from build123d import *

# Parameters (mm, degrees)
SKETCH1_W           = 23
SKETCH1_H           = 60
BOSS_EXTRUDE1_DEPTH = 55
SKETCH2_W           = 55
SKETCH2_H           = 9.5
CUT_EXTRUDE1_DEPTH  = 5
SKETCH3_R           = 1.75
CUT_EXTRUDE2_DEPTH  = 3


with BuildPart() as part:
    # Sketch1 → Boss-Extrude1 (new body)
    with BuildSketch(Plane(origin=(0, 0, 0), x_dir=(0, 0, -1), z_dir=(1, 0, 0))):
        with Locations((11.5, 30)):
            Rectangle(SKETCH1_W, SKETCH1_H)
    extrude(amount=BOSS_EXTRUDE1_DEPTH)

    # Sketch2 → Cut-Extrude1 (cut)
    with BuildSketch(Plane.XY):
        with Locations((27.5, 52.25)):
            Rectangle(SKETCH2_W, SKETCH2_H)
    extrude(amount=-CUT_EXTRUDE1_DEPTH, mode=Mode.SUBTRACT)

    # Sketch3 → Cut-Extrude2 (cut)
    with BuildSketch(Plane.XY.offset(-5)):
        with Locations((7.5, 52.25)):
            Circle(SKETCH3_R)
        with Locations((27.5, 52.25)):
            Circle(SKETCH3_R)
        with Locations((47.5, 52.25)):
            Circle(SKETCH3_R)
    extrude(amount=-CUT_EXTRUDE2_DEPTH, mode=Mode.SUBTRACT)


solid = part.part
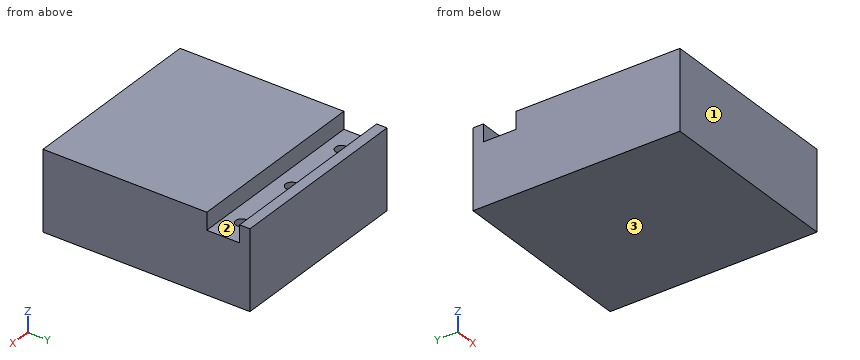
Work out the finished part from the listing and answer in its coordinate system (mm). Face numbers are marked on the shaded views. Round coordinates to 2 decimals unless told otherwise and drop trailing zeros. Write each loop counter-clockwise with the first axis right and the second up, starting at its lowest first coordinate (ties: lowest second). Pieces come first, ordered by that corner, then holes. Notation, with made-up numbers: (33, 58) -> (60, 58) arc R6 ccw to (60, 64) -> close; hole circle Ø2 at (56, 33.5). An arc over 180 degrees is marked (long way). Write each question's results on one line, items separated by ' | '.
Item 1: The mould has two halves that part along Y. Classify the marked faces 1, 2 and 3: +Y half, -Y half, draft (parallel to the pull), parting line (faces both ways), or undercut.
Result set:
face 1: -Y half | face 2: undercut | face 3: draft
Item 2: A cutting plane is placed at A-A, the plane z = -2.75. Determine the outline of the cut face in (x, y).
Result set:
outline: (0, 0) -> (55, 0) -> (55, 47.5) -> (0, 47.5) -> close; (0, 57) -> (55, 57) -> (55, 60) -> (0, 60) -> close
Item 3: A cutting plane is placed at B-B, the plane x = 36. Determine the outline of the cut face in (y, z), plus the area to 3 significant figures.
Result set:
outline: (0, -23) -> (60, -23) -> (60, 0) -> (57, 0) -> (57, -5) -> (47.5, -5) -> (47.5, 0) -> (0, 0) -> close | area: 1,330 mm^2
Item 4: Find the intervals of material crossed by line 1 along Y through (x, z) = (27.5, -5.65); line 2 along Y through (x, z) = (38.5, -2.25), in increasing order. Write a range as [from, to].
Result set:
line 1: [0, 50.5], [54, 60] | line 2: [0, 47.5], [57, 60]
Item 5: A cutting plane is placed at C-C, the plane x = 7.5. Determine the outline of the cut face in (y, z), plus the area to 3 significant figures.
Result set:
outline: (0, -23) -> (60, -23) -> (60, 0) -> (57, 0) -> (57, -5) -> (54, -5) -> (54, -8) -> (50.5, -8) -> (50.5, -5) -> (47.5, -5) -> (47.5, 0) -> (0, 0) -> close | area: 1,320 mm^2
Item 6: Flat-ended cylindrical pins translate along their axes: P1, Ø1.5, axis at x = 7.5, z = -14, coming from the -Y side; P2, Ø1, axis at x = 8, y = 52, coming from the +Z side; P3, Ø4, axis at x = 28, y = 51.5, coming from the +Z side. Find the tip coordinate at first contact, or state that the pin passes through.
Result set:
P1: y = 0 | P2: z = -8 | P3: z = -5
